```python
from build123d import *

# Parameters (mm, degrees)
SCHIZZO1_W                                      = 20
SCHIZZO1_H                                      = 4
ESTRUSIONE_ESTRUSIONE1_DEPTH                    = 20
SCHIZZO2_W                                      = 20
SCHIZZO2_H                                      = 4
ESTRUSIONE_ESTRUSIONE2_DEPTH                    = 20
TAGLIO_ESTRUSIONE2_REACH                        = 6
SCHIZZO7_R                                      = 1.75
RACCORDO1_R                                     = 1
SMUSSO1_SIZE                                    = 2
SMUSSO3_SIZE                                    = 2
CSK_FOR_M3_OVAL_HEAD_MACHINE_SCREW1_D           = 3.4
CSK_FOR_M3_OVAL_HEAD_MACHINE_SCREW1_CSINK_D     = 6.3
CSK_FOR_M3_OVAL_HEAD_MACHINE_SCREW1_CSINK_ANGLE = 90


with BuildPart() as part:
    # Schizzo1 → Estrusione-Estrusione1 (new body)
    with BuildSketch(Plane.XY):
        with Locations((10, 2)):
            Rectangle(SCHIZZO1_W, SCHIZZO1_H)
    extrude(amount=ESTRUSIONE_ESTRUSIONE1_DEPTH)

    # Schizzo2 → Estrusione-Estrusione2 (add)
    with BuildSketch(Plane(origin=(0, 4, 0), x_dir=(1, 0, 0), z_dir=(0, 1, 0))):
        with Locations((10, -18)):
            Rectangle(SCHIZZO2_W, SCHIZZO2_H)
    extrude(amount=ESTRUSIONE_ESTRUSIONE2_DEPTH)

    # Schizzo7 → Taglio-Estrusione2 (cut, up to next)
    with BuildSketch(Plane(origin=(0, 0, 16), x_dir=(-1, 0, 0), z_dir=(0, 0, -1)), mode=Mode.PRIVATE) as taglio_estrusione2_sk1:
        with Locations((-10, 19)):
            Circle(SCHIZZO7_R)
    taglio_estrusione2_tool1 = extrude(taglio_estrusione2_sk1.sketch, amount=-TAGLIO_ESTRUSIONE2_REACH, mode=Mode.PRIVATE) & part.part
    add(taglio_estrusione2_tool1.solids().sort_by_distance((10, 19, 16))[0], mode=Mode.SUBTRACT)
    # Schizzo7 → Taglio-Estrusione2 (cut, up to next)
    with BuildSketch(Plane(origin=(0, 0, 16), x_dir=(-1, 0, 0), z_dir=(0, 0, -1)), mode=Mode.PRIVATE) as taglio_estrusione2_sk2:
        with Locations((-10, 12)):
            Circle(SCHIZZO7_R)
    taglio_estrusione2_tool2 = extrude(taglio_estrusione2_sk2.sketch, amount=-TAGLIO_ESTRUSIONE2_REACH, mode=Mode.PRIVATE) & part.part
    add(taglio_estrusione2_tool2.solids().sort_by_distance((10, 12, 16))[0], mode=Mode.SUBTRACT)

    # Raccordo1
    raccordo1_edges = [part.edges().sort_by_distance(p)[0] for p in [
        (10, 4, 16),
    ]]
    fillet(raccordo1_edges, radius=RACCORDO1_R)

    # Smusso1
    smusso1_edges = [part.edges().sort_by_distance(p)[0] for p in [
        (0, 24, 18),
        (20, 24, 18),
    ]]
    chamfer(smusso1_edges, length=SMUSSO1_SIZE)

    # Smusso3
    smusso3_edges = [part.edges().sort_by_distance(p)[0] for p in [
        (20, 2, 0),
        (0, 2, 0),
    ]]
    chamfer(smusso3_edges, length=SMUSSO3_SIZE)

    # CSK for M3 Oval Head Machine Screw1 (through all)
    with Locations(Plane(origin=(10, 4, 6), x_dir=(0, 0, 1), z_dir=(0, 1, 0))):
        with Locations((0, 0)):
            CounterSinkHole(CSK_FOR_M3_OVAL_HEAD_MACHINE_SCREW1_D / 2, CSK_FOR_M3_OVAL_HEAD_MACHINE_SCREW1_CSINK_D / 2, counter_sink_angle=CSK_FOR_M3_OVAL_HEAD_MACHINE_SCREW1_CSINK_ANGLE)


solid = part.part
```
CAD build for the part. Positions are in the model's coordinates, mm. A direction names the side the tool comes from. Coordinates: 2 decimals unless noted, no trailing zeros. Write each loop counter-clockwise with the first axis right and the second up, starting at its lowest first coordinate (ties: lowest second). Pieces come first, ordered by that corner, then holes.
(1) Cut at C-C, the plane y = 12. List the corners of the cut face in (x, z), and give its area (3 significant figures).
(2) Drill centre lines: probe 1 along Y at (x, z) = (10, 18.85); probe 2 along Z at (x, y) = (19.25, 7.25); probe 3 along X at (y, z) = (1.3, 6). Where is each one in solid material? Low to high.
(3) Flat gauge pins, fed straight in: pin 1 (4 mm diameter, centred on x = 8.5, y = 12, fed in from +Z); pin 2 (3 mm diameter, centred on x = 11, y = 10, fed in from -Z). Where does each tip first touch, or does it go through?
(4) Cut at A-A, the plane z = 6. List the corners of the cut face in (x, y), and give its area (3 significant figures).
(5) Cut at B-B, the plane x = 10. List the corners of the cut face in (y, z), and give its area (3 significant figures).
(6) 3-axis set-ups, long thin cutter, end or side, ignore diameter. For faces 4 (the face through (12, 4, 9)), 5 (the face through (12, 12, 20)): which of +Z, -Z, +X, -X, +Y, -Y reach the whole face in a straight line?
(7) Two-plate mould, pull along Z, no slides. Class faces 1 (the face through (10.228, 20.735, 17.972)), 2 (the face through (8.34, 1.26, 6.37)), 3 (the face through (10, 2, 0)): +Z half, -Z half, draft (parallel to the pull), parting line (faces both ways), or undercut.
(8) Cut at D-D, the plane y = 3.5. List the corners of the cut face in (x, z), and give its area (3 significant figures).
Geometry says:
1. outline: (0, 16) - (8.25, 16) - (8.25, 20) - (0, 20) - close; (11.75, 16) - (20, 16) - (20, 20) - (11.75, 20) - close
1. area: 66.0 mm2
2. probe 1: y = 0 to 10.25, 13.75 to 17.25, 20.75 to 24
2. probe 2: z = 16 to 20
2. probe 3: x = 0 to 8.3, 11.7 to 20
3. pin 1: stops at z = 20
3. pin 2: stops at z = 16
4. outline: (0, 0) - (8.3, 0) - (8.3, 2.55) - (6.85, 4) - (0, 4) - close; (11.7, 0) - (20, 0) - (20, 4) - (13.15, 4) - (11.7, 2.55) - close
4. area: 64.3 mm2
5. outline: (0, 0) - (4, 0) - (4, 2.85) - (2.55, 4.3) - (0, 4.3) - close; (0, 7.7) - (2.55, 7.7) - (4, 9.15) - (4, 15) arc R1 cw to (5, 16) - (10.25, 16) - (10.25, 20) - (0, 20) - close; (13.75, 16) - (17.25, 16) - (17.25, 20) - (13.75, 20) - close; (20.75, 16) - (24, 16) - (24, 20) - (20.75, 20) - close
5. area: 117 mm2
6. face 4: -Z, +X, -X, +Y
6. face 5: +Z, +X, -X, +Y, -Y
7. face 1: draft
7. face 2: undercut
7. face 3: -Z half
8. outline: (0, 2) - (2, 0) - (18, 0) - (20, 2) - (20, 20) - (0, 20) - close; hole circle Ø5.3 at (10, 6)
8. area: 374 mm2
